Here's how the part is built. I have some questions about the finished solid (model axes, mm). A direction names the side the tool comes from. Round coordinates to 2 decimals unless told otherwise and drop trailing zeros. Loops run counter-clockwise (first coordinate to the right, second up) from the corner with the lowest first, then second, coordinate; pieces in that order, holes last. Notation, with made-up numbers: M 38.25,85.5 L 49.25,85.5 A22 ccw 49.25,114.5 Z; hole C 52.5,9 d1. An arc over 180 degrees is marked long. Answer as a JSON object with one key per item and string values.
from build123d import *

# Parameters (mm, degrees)
SKETCH1_R           = 49.75
SKETCH1_R_2         = 3.571875
SKETCH1_R_3         = 5
SKETCH1_R_4         = 3.3
BOSS_EXTRUDE1_DEPTH = 3.175


with BuildPart() as part:
    # Sketch1 → Boss-Extrude1 (new body)
    with BuildSketch(Plane(origin=(0, 0, 0), x_dir=(1, 0, 0), z_dir=(0, 1, 0))):
        with Locations(Location((0, 0, 0), (0, 0, 270))):
            Circle(SKETCH1_R)
        with Locations(Location((0, 36.5125, 0), (0, 0, 270))):
            Circle(SKETCH1_R_2, mode=Mode.SUBTRACT)
        with Locations(Location((0, -36.5125, 0), (0, 0, 270))):
            Circle(SKETCH1_R_2, mode=Mode.SUBTRACT)
        with Locations(Location((30.245937227, -17.4625, 0), (0, 0, 270))):
            Circle(SKETCH1_R_3, mode=Mode.SUBTRACT)
        with Locations(Location((17.4625, 30.245937227, 0), (0, 0, 270))):
            Circle(SKETCH1_R_4, mode=Mode.SUBTRACT)
        with Locations(Location((-30.245937227, 17.4625, 0), (0, 0, 270))):
            Circle(SKETCH1_R_3, mode=Mode.SUBTRACT)
        with Locations(Location((-17.4625, 30.245937227, 0), (0, 0, 270))):
            Circle(SKETCH1_R_4, mode=Mode.SUBTRACT)
        with Locations(Location((-17.4625, -30.245937227, 0), (0, 0, 270))):
            Circle(SKETCH1_R_4, mode=Mode.SUBTRACT)
        with Locations(Location((17.4625, -30.245937227, 0), (0, 0, 270))):
            Circle(SKETCH1_R_4, mode=Mode.SUBTRACT)
        with Locations(Location((30.245937227, 17.4625, 0), (0, 0, 270))):
            Circle(SKETCH1_R_3, mode=Mode.SUBTRACT)
        with Locations(Location((-30.245937227, -17.4625, 0), (0, 0, 270))):
            Circle(SKETCH1_R_3, mode=Mode.SUBTRACT)
        with BuildLine():
            ThreePointArc((-25.748561188, -5.303123397), (0, -26.289), (25.748561188, -5.303123397))
            ThreePointArc((25.748561188, -5.303123397), (27.03087337, -4.059432148), (28.658299321, -4.796030566))
            ThreePointArc((28.658299321, -4.796030566), (45.7152375, 0), (28.658299321, 4.796030566))
            ThreePointArc((28.658299321, 4.796030566), (27.03087337, 4.059432148), (25.748561188, 5.303123397))
            ThreePointArc((25.748561188, 5.303123397), (0, 26.289), (-25.748561188, 5.303123397))
            ThreePointArc((-25.748561188, 5.303123397), (-27.03087337, 4.059432148), (-28.658299321, 4.796030566))
            ThreePointArc((-28.658299321, 4.796030566), (-45.7152375, 0), (-28.658299321, -4.796030566))
            ThreePointArc((-28.658299321, -4.796030566), (-27.03087337, -4.059432148), (-25.748561188, -5.303123397))
        make_face(mode=Mode.SUBTRACT)
    extrude(amount=BOSS_EXTRUDE1_DEPTH)


solid = part.part
Item 1: I want a section at C-C, the plane z = 0. Please give me the cut outline in (x, y) (3 decimals), then the cut area to 3 significant figures.
Resolved:
{"outline": "M -49.75,0 L -45.715,0 L -45.715,3.175 L -49.75,3.175 Z; M 45.715,0 L 49.75,0 L 49.75,3.175 L 45.715,3.175 Z", "area": "25.6 mm²"}
Item 2: Please list where these lines run through material, in increasing order: probe 1 along X at (y, z) = (2.15, 0); probe 2 along X at (y, z) = (2.05, -15.5); probe 3 along X at (y, z) = (2, -5.5). Write a range as from..to.
Resolved:
{"probe 1": "-49.75..-45.72, 45.72..49.75", "probe 2": "-47.27..-34.84, -25.65..-21.23, 21.23..25.65, 34.84..47.27", "probe 3": "-49.45..-43.89, -29.13..-25.71, 25.71..29.13, 43.89..49.45"}
Item 3: On a 3-axis mill with a long thin cutter (end or side, diameter ignored), from which of +Z, -Z, +X, -X, +Y, -Y can I reach the whole of each face in a straight line? I mean faces 4 (the face through (-21, 0, 21)), 5 (the face through (27.057, 1.565, -4.055)). Say none if no direction works.
Resolved:
{"face 4": "+Z, -Z, +X, -X, -Y", "face 5": "+Y, -Y"}
Item 4: I want a section at D-D, the plane x = -38.5. Please give me the cut outline in (y, z) (3 decimals).
Resolved:
{"outline": "M 0,-31.509 L 3.175,-31.509 L 3.175,-8.986 L 0,-8.986 Z; M 0,8.986 L 3.175,8.986 L 3.175,31.509 L 0,31.509 Z"}
Item 5: I want a section at B-B, the plane z = -19. Please give me the cut outline in (x, y) (3 decimals), then the cut area to 3 significant figures.
Resolved:
{"outline": "M -45.979,0 L -35.004,0 L -35.004,3.175 L -45.979,3.175 Z; M -25.488,0 L -18.169,0 L -18.169,3.175 L -25.488,3.175 Z; M 18.169,0 L 25.488,0 L 25.488,3.175 L 18.169,3.175 Z; M 35.004,0 L 45.979,0 L 45.979,3.175 L 35.004,3.175 Z", "area": "116 mm²"}
Item 6: I'm going to push flat-ended pins straight in: pin 1 Ø6 at (x, z) = (-30.25, 17.46) entering from +Y; pin 2 Ø1 at (y, z) = (1, -2) entering from -X; pin 3 Ø1 at (y, z) = (2.5, 8) entering from +X; pin 4 Ø1.5 at (x, y) = (26, 1.5) entering from -Z. Where does each tip first touch, or does it pass through?
Resolved:
{"pin 1": "through", "pin 2": "x = -49.73", "pin 3": "x = 49.18", "pin 4": "z = -42.87"}
Item 7: If we mould it in two halves opening along X, with no side actions, what happens to faces 1 (the face through (-21, 3.175, 21)), 2 (the face through (-28.74, 1.57, 22.23)), 3 (the face through (14.944, 1.565, 47.453))? For each: pulls with the +X half, pulls with the -X half, needs draft (parallel to the pull), parting line crosses it, or undercut.
Resolved:
{"face 1": "needs draft", "face 2": "undercut", "face 3": "parting line crosses it"}
Item 8: I want a section at A-A, the plane x = 0. Please give me the cut outline in (y, z) (3 decimals), then the cut area to 3 significant figures.
Resolved:
{"outline": "M 0,-49.75 L 3.175,-49.75 L 3.175,-40.084 L 0,-40.084 Z; M 0,-32.941 L 3.175,-32.941 L 3.175,-26.289 L 0,-26.289 Z; M 0,26.289 L 3.175,26.289 L 3.175,32.941 L 0,32.941 Z; M 0,40.084 L 3.175,40.084 L 3.175,49.75 L 0,49.75 Z", "area": "104 mm²"}
